For this review, take the finished solid that the model builds, in its own axes (mm). A direction names the side the tool comes from. Coordinates: 2 decimals unless noted, no trailing zeros. Write each loop counter-clockwise with the first axis right and the second up, starting at its lowest first coordinate (ties: lowest second). Pieces come first, ordered by that corner, then holes. Notation, with made-up numbers: (-40, 74) - (0, 74) arc R30 ccw to (0, 109) - close; hole circle Ø3 at (83.25, 33). An arc over 180 degrees is marked (long way). Use one line per item in the form item = value. Start each with the question number.
1) Insertion check: P1, Ø5, axis at x = -11.5, z = -5, coming from the -Y side. The pin has a flat end and moves straight along its axis. Give the tip position at first contact, or say it passes through.
2) We need section A-A (y = 11.5). Give the boundary of the cut face in (x, z).
3) We need section C-C (z = -0.25). Give the boundary of the cut face in (x, y).
4) We need section B-B (x = -37.5). Give the boundary of the cut face in (y, z), plus the area to 3 significant figures.
5) Mouldability with a two-part tool opening along Z and no side actions: class faces 3 (the flat face through (-1, 7, -12.5)), 4 (the flat face through (-1, 0, -12)), 5 (the flat face through (-1, 8, 10.5)) as pulls with the +Z half, pulls with the -Z half, needs draft (parallel to the pull), parting line crosses it, or undercut.
6) For L1, parallel to Z at x = -16.5, y = 5.5; L2, parallel to Y at x = 16, z = -7.25, list the stretches that pass through material, from the lowest coordinate up. Write a range as from..to.
7) Tool access review of faces 1 (the flat face through (-1, 0, 11)), 2 (the flat face through (-1, 8, -10.5)): name each direction out of +Z, -Z, +X, -X, +Y, -Y from which nothing blocks a thin tool from reaching the whole face with its end or side.
```python
from build123d import *

# Parameters (mm, degrees)
CROQUIS1_W              = 115
CROQUIS1_H              = 20.7
CROQUIS1_H_2            = 2.15
SALIENTE_EXTRUIR1_DEPTH = 15
CROQUIS2_W              = 21
CROQUIS2_H              = 13
CORTAR_EXTRUIR1_DEPTH   = 230
SALIENTE_EXTRUIR4_DEPTH = 115


with BuildPart() as part:
    # Croquis1 → Saliente-Extruir1 (new body)
    with BuildSketch(Plane(origin=(0, 0, 0), x_dir=(1, 0, 0), z_dir=(0, 1, 0))):
        Rectangle(CROQUIS1_W, CROQUIS1_H)
        with Locations((0, 11.425)):
            Rectangle(CROQUIS1_W, CROQUIS1_H_2)
        with Locations((0, -11.425)):
            Rectangle(CROQUIS1_W, CROQUIS1_H_2)
    extrude(amount=SALIENTE_EXTRUIR1_DEPTH)

    # Croquis2 → Cortar-Extruir1 (cut)
    with BuildSketch(Plane.ZY.offset(57.5)):
        with Locations((0, 6.5)):
            Rectangle(CROQUIS2_W, CROQUIS2_H)
    extrude(amount=-CORTAR_EXTRUIR1_DEPTH, mode=Mode.SUBTRACT)

    # Croquis11 → Saliente-Extruir4 (add)
    with BuildSketch(Plane.ZY.offset(57.5)):
        Polygon((-10.5, 1.35), (-10.5, 2.55), (-10, 2.55), align=None)
        Polygon((10, 2.55), (10.5, 1.35), (10.5, 2.55), align=None)
    extrude(amount=-SALIENTE_EXTRUIR4_DEPTH)


solid = part.part
```
Determined:
q1.P1 = 13
q2.outline = (-57.5, -12.5) - (57.5, -12.5) - (57.5, -10.5) - (-57.5, -10.5) - close; (-57.5, 10.5) - (57.5, 10.5) - (57.5, 12.5) - (-57.5, 12.5) - close
q3.outline = (-57.5, 13) - (57.5, 13) - (57.5, 15) - (-57.5, 15) - close
q4.outline = (0, -12.5) - (15, -12.5) - (15, 12.5) - (0, 12.5) - (0, 10.5) - (1.35, 10.5) - (2.55, 10) - (2.55, 10.5) - (13, 10.5) - (13, -10.5) - (2.55, -10.5) - (2.55, -10) - (1.35, -10.5) - (0, -10.5) - close
q4.area = 103 mm²
q5.face_3 = pulls with the -Z half
q5.face_4 = needs draft
q5.face_5 = undercut
q6.L1 = -12.5..-10.5, 10.5..12.5
q6.L2 = 13..15
q7.face_1 = +Z, -Z, +X, -X, -Y
q7.face_2 = +X, -X
